Here's how the part is built. I have some questions about the finished solid (model axes, mm). Face numbers are marked on the shaded views. A direction names the side the tool comes from. Coordinates: 2 decimals unless noted, no trailing zeros. Write each loop counter-clockwise with the first axis right and the second up, starting at its lowest first coordinate (ties: lowest second). Pieces come first, ordered by that corner, then holes. Notation, with made-up numbers: (29, 33) - (68, 33) arc R17 cw to (68, 53) - close; hole circle Ø6 at (-38.75, 53.5). An arc over 180 degrees is marked (long way). Answer in a Markdown table with one row per item. Add a question column.
Item 1: We'd pull the mould along Y, two halves only. Please class the marked faces 4, 5 and 6: +Y half, -Y half, draft (parallel to the pull), parting line (faces both ways), or undercut.
Item 2: Imagine slicing it at A-A (z = 96.52). Please give me the cut outline in (x, y), plus the area to 3 significant figures.
Item 3: Imagine slicing it at C-C (z = 76.2). Please give me the cut outline in (x, y).
Item 4: Imagine slicing it at B-B (y = -9). Please give me the cut outline in (x, z), plus the area to 3 significant figures.
Item 5: I'm going to push flat-ended pins straight in: pin 1 (5.5 mm diameter, centred on x = 37.84, z = 90.17, fed in from -Y); pin 2 (3 mm diameter, centred on x = 18.79, z = 96.52, fed in from -Y); pin 3 (6 mm diameter, centred on x = 35, z = 33, fed in from -Y); pin 4 (15.5 mm diameter, centred on x = 27, y = -31, fed in from +Z). Where does each tip first touch, or does it pass through?
Item 6: Imagine slicing it at D-D (x = 30). Please give me the cut outline in (y, z), plus the area to 3 significant figures.
Item 7: If I drill on probe 1 along Z at (x, y) = (73.75, -50.8); probe 2 along X at (y, z) = (-5, 96.52); probe 3 along Z at (x, y) = (74, -31), over which ranges is the centre line in solid material (lowest first)? Write a range as from..to.
Item 8: Which directions (+Z, -Z, +X, -X, +Y, -Y) give clear straight access to the entire face, cutting with the end or side of a thin tool? Please do the marked faces 1, 2 and 3.
from build123d import *

# Parameters (mm, degrees)
BOSS_EXTRUDE1_DEPTH        = 101.6
CUT_EXTRUDE2_START         = -6.35
SKETCH3_W                  = 69.32635313
SKETCH3_H                  = 44.45
CUT_EXTRUDE2_DEPTH         = 58.15
CUT_EXTRUDE3_REACH         = 77.676
SKETCH4_R                  = 12.7
F_10_32_TAPPED_HOLE1_D     = 4.0386
F_10_32_TAPPED_HOLE1_DEPTH = 6.35
F_10_32_TAPPED_HOLE2_D     = 4.0386
F_10_32_TAPPED_HOLE2_DEPTH = 6.35
CUT_EXTRUDE4_DEPTH         = 44.45
CUT_EXTRUDE5_REACH         = 50.644
SKETCH11_R                 = 1.905


with BuildPart() as part:
    # Sketch1 → Boss-Extrude1 (new body)
    with BuildSketch(Plane.XY):
        Polygon((0, 0), (75.67635313, 0), (75.67635313, -63.5), align=None)
        Polygon((17.446481614, -6.35), (69.32635313, -6.35), (69.32635313, -49.882381055), align=None, mode=Mode.SUBTRACT)
    extrude(amount=BOSS_EXTRUDE1_DEPTH)

    # Sketch3 → Cut-Extrude2 (cut, through all)
    with BuildSketch(Plane(origin=(0, 0, 0), x_dir=(1, 0, 0), z_dir=(0, 1, 0)).offset(CUT_EXTRUDE2_START)):
        with Locations((34.663176565, -79.375)):
            Rectangle(SKETCH3_W, SKETCH3_H)
    extrude(amount=-CUT_EXTRUDE2_DEPTH, mode=Mode.SUBTRACT)

    # Sketch4 → Cut-Extrude3 (cut, up to next)
    with BuildSketch(Plane(origin=(75.67635313, 0, 0), x_dir=(0, 0, -1), z_dir=(1, 0, 0)), mode=Mode.PRIVATE) as cut_extrude3_sk1:
        with Locations((-76.2, -31.75)):
            Circle(SKETCH4_R)
    cut_extrude3_tool1 = extrude(cut_extrude3_sk1.sketch, amount=-CUT_EXTRUDE3_REACH, mode=Mode.PRIVATE) & part.part
    add(cut_extrude3_tool1.solids().sort_by_distance((75.676353, -31.75, 76.2))[0], mode=Mode.SUBTRACT)

    # #10-32 Tapped Hole1
    with Locations(Plane(origin=(75.67635313, -50.8, 85.725), x_dir=(0, 1, 0), z_dir=(1, 0, 0))):
        with Locations((0, 0), (0, -19.05), (38.1, 0), (38.1, -19.05)):
            Hole(F_10_32_TAPPED_HOLE1_D / 2, depth=F_10_32_TAPPED_HOLE1_DEPTH)

    # #10-32 Tapped Hole2
    with Locations(Plane(origin=(0, 0, 0), x_dir=(1, 0, 0), z_dir=(0, 1, 0))):
        with Locations((56.888176565, -96.52), (37.838176565, -90.17), (18.788176565, -96.52)):
            Hole(F_10_32_TAPPED_HOLE2_D / 2, depth=F_10_32_TAPPED_HOLE2_DEPTH)

    # Sketch10 → Cut-Extrude4 (cut)
    with BuildSketch(Plane(origin=(0, 0, 0), x_dir=(-1, 0, 0), z_dir=(0, 0, -1))):
        Polygon((-75.67635313, -55.210663713), (-9.878846301, 0), (-75.67635313, 0), align=None)
    extrude(amount=-CUT_EXTRUDE4_DEPTH, mode=Mode.SUBTRACT)

    # Sketch11 → Cut-Extrude5 (cut, up to next)
    with BuildSketch(Plane(origin=(0, 0, 0), x_dir=(0.766044443, -0.64278761, 0), z_dir=(-0.64278761, -0.766044443, 0)), mode=Mode.PRIVATE) as cut_extrude5_sk1:
        with Locations((54.719463006, 37.719)):
            Circle(SKETCH11_R)
    cut_extrude5_tool1 = extrude(cut_extrude5_sk1.sketch, amount=-CUT_EXTRUDE5_REACH, mode=Mode.PRIVATE) & part.part
    add(cut_extrude5_tool1.solids().sort_by_distance((41.917541, -35.172993, 37.719))[0], mode=Mode.SUBTRACT)
    # Sketch11 → Cut-Extrude5 (cut, up to next)
    with BuildSketch(Plane(origin=(0, 0, 0), x_dir=(0.766044443, -0.64278761, 0), z_dir=(-0.64278761, -0.766044443, 0)), mode=Mode.PRIVATE) as cut_extrude5_sk2:
        with Locations((86.088463006, 37.719)):
            Circle(SKETCH11_R)
    cut_extrude5_tool2 = extrude(cut_extrude5_sk2.sketch, amount=-CUT_EXTRUDE5_REACH, mode=Mode.PRIVATE) & part.part
    add(cut_extrude5_tool2.solids().sort_by_distance((65.947589, -55.336597, 37.719))[0], mode=Mode.SUBTRACT)
    # Sketch11 → Cut-Extrude5 (cut, up to next)
    with BuildSketch(Plane(origin=(0, 0, 0), x_dir=(0.766044443, -0.64278761, 0), z_dir=(-0.64278761, -0.766044443, 0)), mode=Mode.PRIVATE) as cut_extrude5_sk3:
        with Locations((54.719463006, 6.35)):
            Circle(SKETCH11_R)
    cut_extrude5_tool3 = extrude(cut_extrude5_sk3.sketch, amount=-CUT_EXTRUDE5_REACH, mode=Mode.PRIVATE) & part.part
    add(cut_extrude5_tool3.solids().sort_by_distance((41.917541, -35.172993, 6.35))[0], mode=Mode.SUBTRACT)
    # Sketch11 → Cut-Extrude5 (cut, up to next)
    with BuildSketch(Plane(origin=(0, 0, 0), x_dir=(0.766044443, -0.64278761, 0), z_dir=(-0.64278761, -0.766044443, 0)), mode=Mode.PRIVATE) as cut_extrude5_sk4:
        with Locations((86.088463006, 6.35)):
            Circle(SKETCH11_R)
    cut_extrude5_tool4 = extrude(cut_extrude5_sk4.sketch, amount=-CUT_EXTRUDE5_REACH, mode=Mode.PRIVATE) & part.part
    add(cut_extrude5_tool4.solids().sort_by_distance((65.947589, -55.336597, 6.35))[0], mode=Mode.SUBTRACT)


solid = part.part
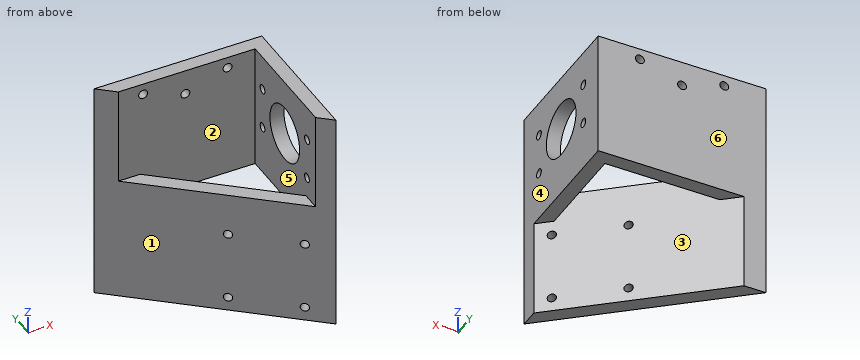
Here are the results:
| question | item | result |
|---|---|---|
| 1 | face 4 | draft |
| 1 | face 5 | undercut |
| 1 | face 6 | +Y half |
| 2 | outline | (0, 0) - (7.57, -6.35) - (16.77, -6.35) - (16.77, 0) - close; (20.81, -6.35) - (54.87, -6.35) - (54.87, 0) - (20.81, 0) - close; (58.91, -6.35) - (69.33, -6.35) - (69.33, -58.17) - (75.68, -63.5) - (75.68, 0) - (58.91, 0) - close |
| 2 | area | 751 mm2 |
| 3 | outline | (0, 0) - (7.57, -6.35) - (69.33, -6.35) - (69.33, -19.05) - (75.68, -19.05) - (75.68, 0) - close; (69.33, -58.17) - (75.68, -63.5) - (75.68, -44.45) - (69.33, -44.45) - close |
| 4 | outline | (10.73, 0) - (20.6, 0) - (20.6, 57.15) - (10.73, 57.15) - close; (69.33, 44.45) - (75.68, 44.45) - (75.68, 101.6) - (69.33, 101.6) - close |
| 4 | area | 927 mm2 |
| 5 | pin 1 | stops at y = -6.35 |
| 5 | pin 2 | passes through |
| 5 | pin 3 | stops at y = -31.89 |
| 5 | pin 4 | stops at z = 57.15 |
| 6 | outline | (-25.17, 0) - (-16.88, 0) - (-16.88, 57.15) - (-25.17, 57.15) - close; (-6.35, 44.45) - (0, 44.45) - (0, 101.6) - (-6.35, 101.6) - close |
| 6 | area | 837 mm2 |
| 7 | probe 1 | z = 44.45..64.66, 68.69..83.71, 87.74..101.6 |
| 7 | probe 2 | x = 5.96..16.77, 20.81..54.87, 58.91..75.68 |
| 7 | probe 3 | z = 44.45..63.52, 88.88..101.6 |
| 8 | face 1 | +Z, -Z, -X, -Y |
| 8 | face 2 | +Z |
| 8 | face 3 | -Z |
